Work out the finished part from the listing and answer in its coordinate system (mm). A direction names the side the tool comes from. Coordinates: 2 decimals unless noted, no trailing zeros. Loops run counter-clockwise (first coordinate to the right, second up) from the corner with the lowest first, then second, coordinate; pieces in that order, holes last. Notation, with made-up numbers: M 68.25,40 L 100.25,40 A21 cw 100.25,69 Z; hole C -10.5,17 d1. An arc over 180 degrees is marked long. Write each question's results on one line, items separated by ' | '.
```python
from build123d import *

# Parameters (mm, degrees)
SKETCH2_R           = 2.25
BOSS_EXTRUDE1_DEPTH = 25
BOSS_EXTRUDE3_DEPTH = 4


with BuildPart() as part:
    # Sketch2 → Boss-Extrude1 (new body)
    with BuildSketch(Plane(origin=(0, 0, 0), x_dir=(1, 0, 0), z_dir=(0, 1, 0))):
        with Locations(Location((0, 0, 0), (0, 0, 270))):
            Circle(SKETCH2_R)
    extrude(amount=-BOSS_EXTRUDE1_DEPTH)

    # Sketch3 → Boss-Extrude3 (add)
    with BuildSketch(Plane(origin=(0, 0, 0), x_dir=(1, 0, 0), z_dir=(0, 1, 0))):
        Polygon((0, 3.75277675), (-3.25, 1.876388375), (-3.25, -1.876388375), (0, -3.75277675), (3.25, -1.876388375), (3.25, 1.876388375), align=None)
    extrude(amount=-BOSS_EXTRUDE3_DEPTH)

    # Sketch5 → Cut-Revolve2 (revolve, cut)
    with BuildSketch(Plane(origin=(0, 0, 0), x_dir=(0, 0, -1), z_dir=(1, 0, 0))):
        Polygon((3.25277675, 0), (3.75277675, 0), (3.75277675, -0.5), align=None)
    revolve(axis=Axis((0, 0, 0), (0, -1, 0)), mode=Mode.SUBTRACT)


solid = part.part
```
1) Straight lines are drawn through the part: probe 1 along Z at (x, y) = (1.25, -10.75); probe 2 along Y at (x, z) = (-1.75, -2). For each, find the intervals that lie inside material, in ascending order. Write a range as [from, to].
Check result:
probe 1: [-1.87, 1.87] | probe 2: [-4, 0]
2) Given pin 1 Ø1.5 at (x, y) = (2, -9.5) entering from +Z; pin 2 Ø1 at (x, y) = (1.5, -3) entering from +Z, each flat-ended and moving along its own axis, determine where each tip first touches the part or whether it passes through.
Check result:
pin 1: z = 1.87 | pin 2: z = 3.18
3) Which of the six approach directions +Z, -Z, +X, -X, +Y, -Y give full straight-line access (tool end or side, diameter ignored) to faces 1 (the face through (0.676, -14.353, 2.146)), 2 (the face through (-2.932, -0.138, 1.702))?
Check result:
face 1: -Y | face 2: +Z, -X, +Y
4) Find section A-A, the plane y = -2.5. Give the vertices of the cut face in (x, z), and give its area (3 significant figures).
Check result:
outline: M -3.25,-1.88 L 0,-3.75 L 3.25,-1.88 L 3.25,1.88 L 0,3.75 L -3.25,1.88 Z | area: 36.6 mm^2
5) Find section B-B, the plane y = -6. Give the vertices of the cut face in (x, z).
Check result:
outline: C 0,0 d4.5
